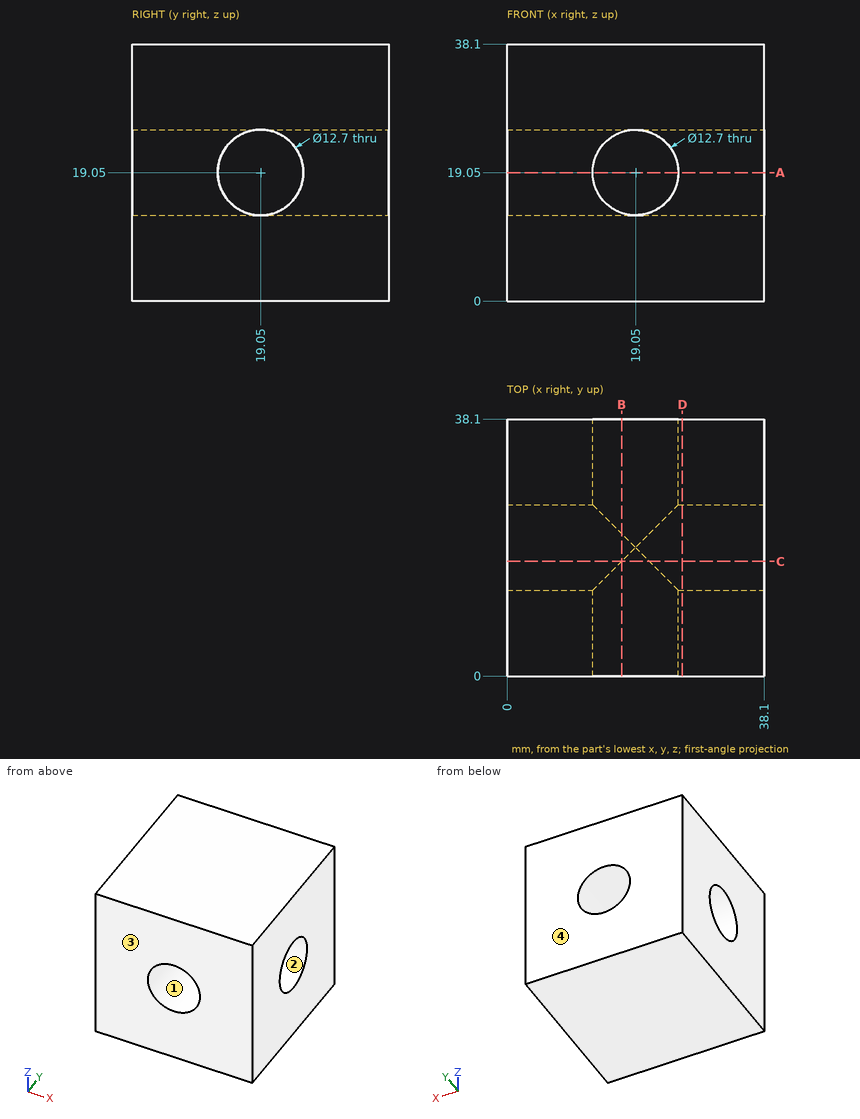
For this review, use the dimensioned drawing (mm, ordinates from the lowest corner) and the shaded views. Coordinates: 2 decimals unless noted, no trailing zeros. Write each loop counter-clockwise with the first axis right and the second up, starting at its lowest first coordinate (ties: lowest second). Pieces come first, ordered by that corner, then holes. Notation, with made-up numbers: (14.5, 21.25) - (32.5, 21.25) arc R21 cw to (32.5, 34.25) - close; hole circle Ø10 at (-35, 78). An arc over 180 degrees is marked (long way). Answer as a JSON object with one key per item and string values. Group by question number.
1. Add section D-D (x = 26). Give the boundary of the cut face in (y, z), plus the area to 3 significant figures.
2. Add section B-B (x = 17). Give the boundary of the cut face in (y, z).
3. Mouldability with a two-part tool opening along Y and no side actions: class the marked faces 1, 2, 3 and 4 as pulls with the +Y half, pulls with the -Y half, needs draft (parallel to the pull), parting line crosses it, or undercut.
4. Add section A-A (z = 19.05). Give the boundary of the cut face in (x, y).
5. To check wall thickness, follow probe 1 along Z at (x, y) = (19, 13); probe 2 along Y at (x, z) = (7, 24). State the ranges of each line that lie inside material, in increasing order.
6. Clearance check with a flat-ended pin moving along its axis: pin 1 Ø11.5 at (x, z) = (19.05, 19.05) entering from +Y. State where the tip first meets the part, or that it passes through.
Findings:
{
 "1": {"outline": "(0, 0) - (38.1, 0) - (38.1, 38.1) - (0, 38.1) - close; hole circle Ø12.7 at (19.05, 19.05)", "area": "1,320 mm²"},
 "2": {"outline": "(0, 0) - (38.1, 0) - (38.1, 13.04) - (21.1, 13.04) arc R6.35 cw to (17, 13.04) - (0, 13.04) - close; (0, 25.06) - (17, 25.06) arc R6.35 cw to (21.1, 25.06) - (38.1, 25.06) - (38.1, 38.1) - (0, 38.1) - close"},
 "3": {"face 1": "needs draft", "face 2": "undercut", "face 3": "pulls with the -Y half", "face 4": "pulls with the +Y half"},
 "4": {"outline": "(0, 0) - (12.7, 0) - (12.7, 12.7) - (0, 12.7) - close; (0, 25.4) - (12.7, 25.4) - (12.7, 38.1) - (0, 38.1) - close; (25.4, 0) - (38.1, 0) - (38.1, 12.7) - (25.4, 12.7) - close; (25.4, 25.4) - (38.1, 25.4) - (38.1, 38.1) - (25.4, 38.1) - close"},
 "5": {"probe 1": "0 to 12.7, 25.4 to 38.1", "probe 2": "0 to 15.07, 23.03 to 38.1"},
 "6": {"pin 1": "through"}
}
